Geometry: final body of the model. Coordinates: model frame, mm. A direction names the side the tool comes from. Give positions to 0.01 mm unless a question says otherwise; leave off trailing zeros. Write each loop counter-clockwise with the first axis right and the second up, starting at its lowest first coordinate (ties: lowest second). Pieces come first, ordered by that corner, then holes.
```python
from build123d import *

# Parameters (mm, degrees)
F0_W     = 88
F0_H     = 64
F0_W_2   = 86
F0_H_2   = 62
F1_DEPTH = 17.5
F0_W_3   = 53
F0_H_3   = 57
F0_W_4   = 26
F0_H_4   = 52
F0_R     = 1.05
F0_R_2   = 2
F0_R_3   = 1.1
F2_DEPTH = 1
F3_DEPTH = 5
F4_R     = 1.8396307345


with BuildPart() as f1:
    # F0 (on Top) → F1 (new body)
    with BuildSketch(Plane.XY):
        Rectangle(F0_W, F0_H)
        Rectangle(F0_W_2, F0_H_2, mode=Mode.SUBTRACT)
    extrude(amount=F1_DEPTH)

    # F0 (on Top) → F2 (join)
    with BuildSketch(Plane.XY):
        Rectangle(F0_W_2, F0_H_2)
        with Locations((-14.4680143297, -0.051781863)):
            Rectangle(F0_W_3, F0_H_3, mode=Mode.SUBTRACT)
        with Locations((28.3339827135, -0.5997789651)):
            Rectangle(F0_W_4, F0_H_4, mode=Mode.SUBTRACT)
        with Locations((-14.4680143297, -0.051781863)):
            Rectangle(F0_W_3, F0_H_3)
        with Locations((-37.9180143297, -22.001781863)):
            Circle(F0_R, mode=Mode.SUBTRACT)
        with Locations((8.9319856703, -22.551781863)):
            Circle(F0_R_2, mode=Mode.SUBTRACT)
        with Locations((5.9319856703, 22.348218137)):
            Circle(F0_R_3, mode=Mode.SUBTRACT)
        with Locations((28.3339827135, -0.5997789651)):
            Rectangle(F0_W_4, F0_H_4)
    extrude(amount=F2_DEPTH)

    # F0 (on Top) → F3 (join)
    with BuildSketch(Plane.XY):
        with Locations((8.9319856703, -22.551781863)):
            Circle(F0_R_2)
        with Locations((-37.9180143297, -22.001781863)):
            Circle(F0_R)
        with Locations((5.9319856703, 22.348218137)):
            Circle(F0_R_3)
    extrude(amount=F3_DEPTH)

    # F4
    f4_edges = [f1.edges().sort_by_distance(p)[0] for p in [
        (-44, -32, 8.75),
        (44, -32, 8.75),
        (44, 32, 8.75),
        (-44, 32, 8.75),
        (0, -32, 0),
        (-44, 0, 0),
        (0, 32, 0),
        (44, 0, 0),
        (-43, -31, 9.25),
        (-43, 31, 9.25),
        (43, 31, 9.25),
        (43, -31, 9.25),
    ]]
    fillet(f4_edges, radius=F4_R)


solid = f1.part
```
Item 1: Reachability of faces 1 (the face through (-1, 32, 10)), 2 (the face through (6, 22, 5)) from +Z, -Z, +X, -X, +Y, -Y: full face, straight path, thin tool, end or side. Return the list, or none.
Found:
face 1: +Z, -Z, +X, -X, +Y
face 2: +Z
Item 2: Pin query (flat end, axial travel): pin 1 Ø0.6 at (x, y) = (-37.5, -21.5) entering from +Z; pin 2 Ø6 at (x, y) = (-21.5, -8.5) entering from +Z. Return the tip coordinate at first contact, or that it passes through.
Found:
pin 1: stops at z = 5
pin 2: stops at z = 1
Item 3: Section A-A, the plane z = 14. Return the cut outline in (x, y).
Found:
outline: (-44, -30.16) arc R1.84 ccw to (-42.16, -32) - (42.16, -32) arc R1.84 ccw to (44, -30.16) - (44, 30.16) arc R1.84 ccw to (42.16, 32) - (-42.16, 32) arc R1.84 ccw to (-44, 30.16) - close; hole (-43, -29.16) arc R1.84 ccw to (-41.16, -31) - (41.16, -31) arc R1.84 ccw to (43, -29.16) - (43, 29.16) arc R1.84 ccw to (41.16, 31) - (-41.16, 31) arc R1.84 ccw to (-43, 29.16) - close
Item 4: Section B-B, the plane y = 25.5. Return the cut outline in (x, z), plus the area to 3 significant figures.
Found:
outline: (-44, 1.84) arc R1.84 ccw to (-42.16, 0) - (42.16, 0) arc R1.84 ccw to (44, 1.84) - (44, 17.5) - (43, 17.5) - (43, 1) - (-43, 1) - (-43, 17.5) - (-44, 17.5) - close
area: 120 mm2
Item 5: Pull-direction query (X, two-part tool) for faces 3 (the face through (44, 0, 10)), 4 (the face through (-1, -32, 10)), 5 (the face through (-38.05, -20.96, 2.97)); classes: +X half, -X half, draft (parallel to the pull), parting line (faces both ways), or undercut.
Found:
face 3: +X half
face 4: draft
face 5: undercut
Item 6: Line query: L1, parallel to X at y = 22.5, z = 12; L2, parallel to Y at x = -19.5, z = 8.75; L3, parallel to X at y = 23, z = 2. Output: solid intervals per line, ascending.
Found:
L1: x = -44 to -43, 43 to 44
L2: y = -32 to -31, 31 to 32
L3: x = -44 to -43, 5.05 to 6.82, 43 to 44
Item 7: Section C-C, the plane x = 19. Return the cut outline in (y, z).
Found:
outline: (-32, 1.84) arc R1.84 ccw to (-30.16, 0) - (30.16, 0) arc R1.84 ccw to (32, 1.84) - (32, 17.5) - (31, 17.5) - (31, 1) - (-31, 1) - (-31, 17.5) - (-32, 17.5) - close
